Print and shaded views of the part. All mm, measured from the part's lowest x, y and z. A direction names the side the tool comes from. Give positions to 0.01 mm unless a question says otherwise; leave off trailing zeros. Loops run counter-clockwise (first coordinate to the right, second up) from the corner with the lowest first, then second, coordinate; pieces in that order, holes last.
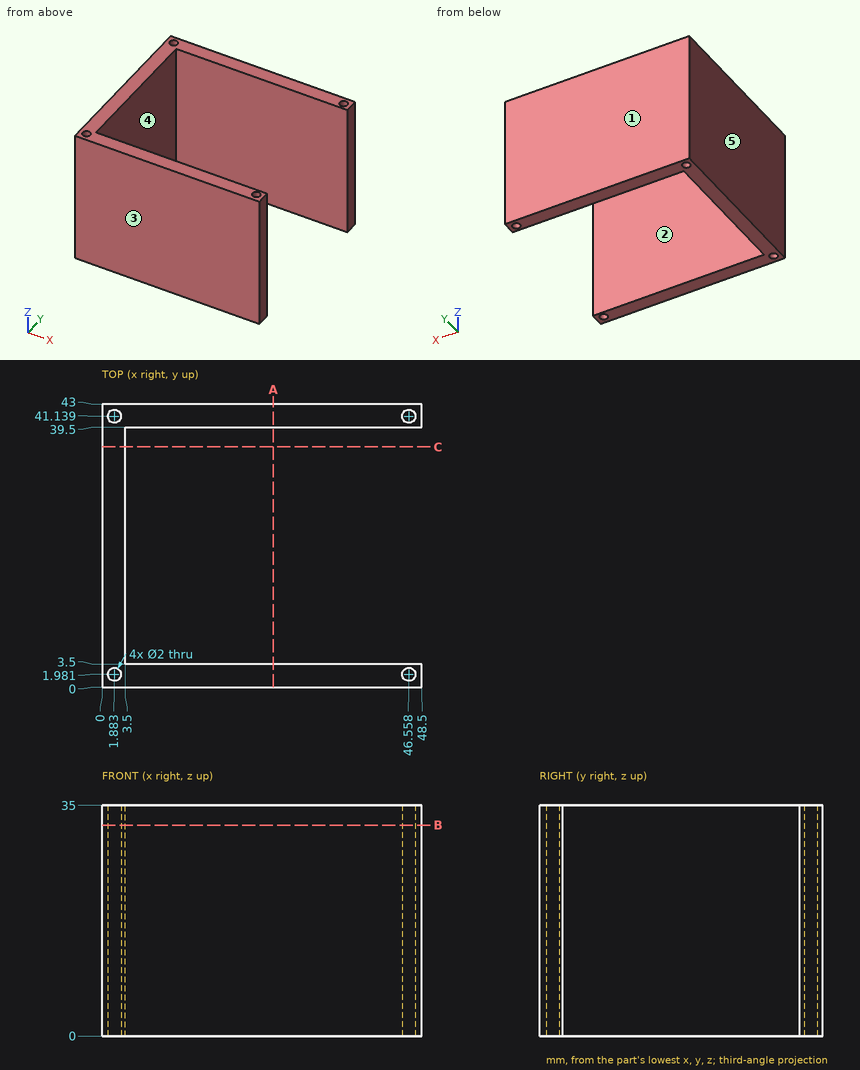
1. Saw through at B-B, the plane z = 32. List the corners of the cut face in (x, y), and give its area (3 significant figures).
Responses:
outline: (0, 0) - (48.5, 0) - (48.5, 3.5) - (3.5, 3.5) - (3.5, 39.5) - (48.5, 39.5) - (48.5, 43) - (0, 43) - close; hole circle Ø2 at (1.88, 1.98); hole circle Ø2 at (1.88, 41.14); hole circle Ø2 at (46.56, 1.98); hole circle Ø2 at (46.56, 41.14)
area: 453 mm2
2. Drop a flat-ended pin along its axis: pin 1 (17.5 mm diameter, centred on y = 16, z = 23.5, fed in from +X). Give the stop position or say it passes through.
Responses:
pin 1: stops at x = 3.5
3. Probe line 1 along X through (y, z) = (41, 17); line 2 along X through (y, z) = (2, 33); line 3 along Y through (x, z) = (16, 17). List the from-to ranges inside material, lowest first.
Responses:
line 1: x = 0 to 0.89, 2.87 to 45.57, 47.55 to 48.5
line 2: x = 0 to 0.88, 2.88 to 45.56, 47.56 to 48.5
line 3: y = 0 to 3.5, 39.5 to 43
4. Pull direction Y, two halves, no side cores. Call the marked faces 1, 2 and 3: released by +Y, released by -Y, zero draft, split by the parting line, or undercut.
Responses:
face 1: released by +Y
face 2: undercut
face 3: released by -Y
5. Tool access for the marked faces 4 and 5: list every direction of +Z, -Z, +X, -X, +Y, -Y with a clear straight run to the whole face (end or side of a thin tool).
Responses:
face 4: +Z, -Z, +X
face 5: +Z, -Z, -X, +Y, -Y
6. Saw through at C-C, the plane y = 36.5. List the corners of the cut face in (x, z).
Responses:
outline: (0, 0) - (3.5, 0) - (3.5, 35) - (0, 35) - close
7. Saw through at A-A, the plane x = 26. List the corners of the cut face in (y, z), and give its area (3 significant figures).
Responses:
outline: (0, 0) - (3.5, 0) - (3.5, 35) - (0, 35) - close; (39.5, 0) - (43, 0) - (43, 35) - (39.5, 35) - close
area: 245 mm2
